```python
from build123d import *

# Parameters (mm, degrees)
ENL_V_MAT_EXTRU_1_DEPTH = 1.2
CHANFREIN1_SIZE         = 0.15


with BuildPart() as part:
    # Esquisse1 → Révolution1 (revolve)
    with BuildSketch(Plane.XY, mode=Mode.PRIVATE) as r_volution1_sk:
        with BuildLine():
            Line((1.5, -5.5), (1, -6))
            Line((1, -6), (0, -6))
            Line((0, -6), (0, 0))
            Line((0, 0), (2.858578644, 0))
            ThreePointArc((2.858578644, 0), (2.98923494, -0.087301746), (2.958578644, -0.241421356))
            Line((2.958578644, -0.241421356), (1.5, -1.7))
            Line((1.5, -1.7), (1.5, -5.5))
        make_face()
    revolve(r_volution1_sk.sketch.rotate(Axis((0, 6.972972973, 0), (0, -1, 0)), 90), axis=Axis((0, 6.972972973, 0), (0, -1, 0)))

    # Esquisse2 → Enlèv. mat.-Extru.1 (cut)
    with BuildSketch(Plane(origin=(0, 0, 0), x_dir=(1, 0, 0), z_dir=(0, 1, 0))):
        Polygon((-1.154700538, 0), (-0.577350269, -1), (0.577350269, -1), (1.154700538, 0), (0.577350269, 1), (-0.577350269, 1), align=None)
    extrude(amount=-ENL_V_MAT_EXTRU_1_DEPTH, mode=Mode.SUBTRACT)

    # Chanfrein1
    chanfrein1_edges = [part.edges().sort_by_distance(p)[0] for p in [
        (-0.8660254037844384, 0, -0.49999999999999983),
        (-0.8660254037844384, 0, 0.5),
        (0, 0, 1),
        (0.866025403784439, 0, 0.5),
        (0.866025403784439, 0, -0.5000000000000004),
        (0, 0, -1),
    ]]
    chamfer(chanfrein1_edges, length=CHANFREIN1_SIZE)


solid = part.part
```
Geometry check sheet. Reference: the model listing, model coordinates, mm. A direction names the side the tool comes from. Give positions to 0.01 mm unless a question says otherwise; leave off trailing zeros. Order: outer loops, then holes, each group sorted by start corner. A loop starts at its lowest first (then second) coordinate and runs counter-clockwise, first axis right, second up. Notation, with made-up numbers: (-18, -36) - (-13, -36) arc R20 ccw to (-13, -6) - close; hole circle Ø10 at (30.25, 40). An arc over 180 degrees is marked (long way). Answer in a Markdown table with one row per item. Add a question column.
Q1. Mould release check, pull along X, two halves, no side actions. Record for faces 1 (the cylindrical face through (-0.45, -3.63, 1.43)), 2 (the flat face through (0, -6, 0)), 3 (the flat face through (0.87, -0.67, -0.49)): pulls with the +X half, pulls with the -X half, needs draft (parallel to the pull), parting line crosses it, or undercut.
Q2. Material ranges on probe 1 along Z at (x, y) = (-0.5, -0.25); probe 2 along X at (y, z) = (-2.75, 0); probe 3 along Z at (x, y) = (-0.75, -3.75), recorded low to high. Write a range as from..to.
Q3. Cross-section at B-B, the plane y = -4.5. Enter the section's corners in (x, z).
Q4. Gauge pin test, flat ends, axial feed: pin 1 (1.5 mm diameter, centred on y = -5, z = 1.5, fed in from +X); pin 2 (1 mm diameter, centred on y = -1, z = 0, fed in from +X); pin 3 (2 mm diameter, centred on x = -1.5, y = -1.5, fed in from +Z). Record the tip position at first contact, or that the pin passes through.
Q5. Tool access check on faces 4 (the flat face through (0, -1, 1)), 5 (the flat face through (1, 0, -1)). Record the directions out of +Z, -Z, +X, -X, +Y, -Y that give a thin tool (end or side, any length) a straight path to the whole face; none if there is none.
Q6. Cross-section at A-A, the plane x = 0. Enter the section's corners in (y, z).
Check values:
| question | item | result |
|---|---|---|
| 1 | face 1 | parting line crosses it |
| 1 | face 2 | needs draft |
| 1 | face 3 | undercut |
| 2 | probe 1 | z = -2.91..-1, 1..2.91 |
| 2 | probe 2 | x = -1.5..1.5 |
| 2 | probe 3 | z = -1.3..1.3 |
| 3 | outline | circle Ø3 at (0, 0) |
| 4 | pin 1 | stops at x = 1.3 |
| 4 | pin 2 | stops at x = 2.7 |
| 4 | pin 3 | stops at z = 2.37 |
| 5 | face 4 | +Y |
| 5 | face 5 | +Z, -Z, +X, -X, +Y |
| 6 | outline | (-6, -1) - (-5.5, -1.5) - (-1.7, -1.5) - (-0.24, -2.96) arc R0.14 ccw to (0, -2.86) - (0, -1.15) - (-0.15, -1) - (-1.2, -1) - (-1.2, 1) - (-0.15, 1) - (0, 1.15) - (0, 2.86) arc R0.14 ccw to (-0.24, 2.96) - (-1.7, 1.5) - (-5.5, 1.5) - (-6, 1) - close |
